from build123d import *

# Parameters (mm, degrees)
SKETCH1_W           = 260
SKETCH1_H           = 47
BOSS_EXTRUDE1_DEPTH = 6
SKETCH3_W           = 6
SKETCH3_H           = 17.5
SKETCH3_H_2         = 7.5
CUT_EXTRUDE1_DEPTH  = 7
SKETCH4_W           = 53
SKETCH4_H           = 6
CUT_EXTRUDE2_DEPTH  = 7
SKETCH5_W           = 14
SKETCH5_H           = 7.5
SKETCH5_W_2         = 6
SKETCH5_H_2         = 12
CUT_EXTRUDE3_DEPTH  = 7
FILLET1_R           = 2


with BuildPart() as part:
    # Sketch1 → Boss-Extrude1 (new body)
    with BuildSketch(Plane.XY):
        Rectangle(SKETCH1_W, SKETCH1_H)
    extrude(amount=-BOSS_EXTRUDE1_DEPTH)

    # Sketch3 → Cut-Extrude1 (cut, through all)
    with BuildSketch(Plane.XY):
        with Locations((-127, 14.75)):
            Rectangle(SKETCH3_W, SKETCH3_H)
        Polygon((-124, -6), (-130, -6), (-130, -23.5), (-124, -23.5), (-124, -17.5), (-124, -10), align=None)
        with Locations((-121, -13.75)):
            Rectangle(SKETCH3_W, SKETCH3_H_2)
    cut_extrude1 = extrude(amount=-CUT_EXTRUDE1_DEPTH, mode=Mode.SUBTRACT)

    # Mirror1: Cut-Extrude1 across plane
    add(cut_extrude1.mirror(Plane(origin=(0, 0, 0), x_dir=(0, 0, 1), z_dir=(1, 0, 0))), mode=Mode.SUBTRACT)

    # Sketch4 → Cut-Extrude2 (cut, through all)
    with BuildSketch(Plane.XY):
        Polygon((-118, -17.5), (-124, -17.5), (-124, -23.5), (-71, -23.5), (-71, -17.5), align=None)
        with Locations((-32.5, -20.5)):
            Rectangle(SKETCH4_W, SKETCH4_H)
        with Locations((32.5, -20.5)):
            Rectangle(SKETCH4_W, SKETCH4_H)
        Polygon((71, -17.5), (71, -23.5), (124, -23.5), (124, -17.5), (118, -17.5), align=None)
    cut_extrude2 = extrude(amount=-CUT_EXTRUDE2_DEPTH, mode=Mode.SUBTRACT)

    # Mirror2: Cut-Extrude2 across plane
    add(cut_extrude2.mirror(Plane.ZX), mode=Mode.SUBTRACT)

    # Sketch5 → Cut-Extrude3 (cut, through all)
    with BuildSketch(Plane.XY):
        with Locations((-117, 13.75)):
            Rectangle(SKETCH5_W, SKETCH5_H)
        with Locations((-107, 0)):
            Rectangle(SKETCH5_W_2, SKETCH5_H_2)
    extrude(amount=-CUT_EXTRUDE3_DEPTH, mode=Mode.SUBTRACT)

    # Fillet1
    fillet1_edges = [part.edges().sort_by_distance(p)[0] for p in [
        (-110, 10, -3),
    ]]
    fillet(fillet1_edges, radius=FILLET1_R)


solid = part.part
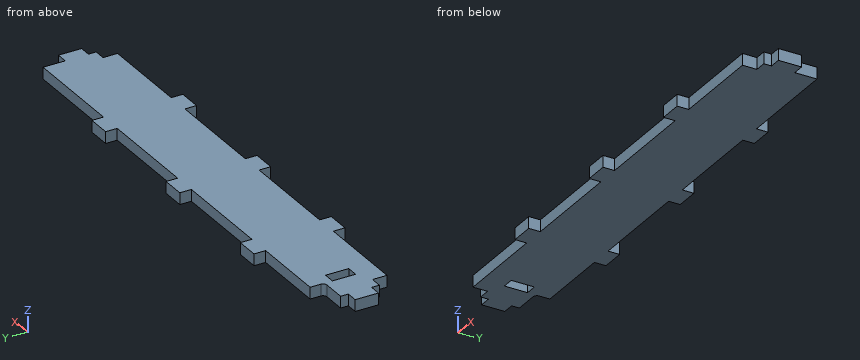
Model file for the job. Use its own axes, mm. Give positions to 0.01 mm unless a question says otherwise; leave off trailing zeros. Write each loop counter-clockwise with the first axis right and the second up, starting at its lowest first coordinate (ties: lowest second). Pieces come first, ordered by that corner, then holes. Notation, with made-up numbers: (43, 13) - (72, 13) arc R12 cw to (72, 22) - close; hole circle Ø6 at (69, -39.75). An arc over 180 degrees is marked (long way). Answer as CSV lines item,"result".
1. Drill centre lines: L1, parallel to X at y = 20, z = -0.75; L2, parallel to X at y = 0, z = -2.1; L3, parallel to Y at x = 106, z = -4.6. Where is each one in solid material? Low to high. Write a range as [from, to].
Responses:
L1,"x = [-71, -59], [-6, 6], [59, 71]"
L2,"x = [-130, -110], [-104, 130]"
L3,"y = [-17.5, 17.5]"
2. Band-saw the part on B-B (y = -13). Write the cut outline in (x, z), and give its area (3 significant figures).
Responses:
outline,"(-118, -6) - (118, -6) - (118, 0) - (-118, 0) - close"
area,"1,420 mm2"
3. Band-saw the part on A-A (x = -79). Write the cut outline in (y, z), and give its area (3 significant figures).
Responses:
outline,"(-17.5, -6) - (17.5, -6) - (17.5, 0) - (-17.5, 0) - close"
area,"210 mm2"
4. Pin check, flat tips, straight feed: pin 1 (3 mm diameter, centred on x = -50.5, z = -5.5, fed in from +Y); pin 2 (3 mm diameter, centred on y = -19.5, z = -2.5, fed in from -X); pin 3 (1.8 mm diameter, centred on x = -86.5, z = -4, fed in from -Y). Stop position of each tip, or through.
Responses:
pin 1,"stops at y = 17.5"
pin 2,"stops at x = -71"
pin 3,"stops at y = -17.5"
